Read the model definition and answer for the solid it produces. Units are mm, in the model's axes. Round coordinates to 2 decimals unless told otherwise and drop trailing zeros. Write each loop counter-clockwise with the first axis right and the second up, starting at its lowest first coordinate (ties: lowest second). Pieces come first, ordered by that corner, then holes. Notation, with made-up numbers: (45, 10) - (86, 10) arc R29 ccw to (86, 31) - close; hole circle Ø2 at (2, 50). An arc over 180 degrees is marked (long way). Answer as CSV lines item,"result". Start each with the question number.
1) Each of these flat-tipped pins is pushed along its axis until it touches: pin 1 (1 mm diameter, centred on x = 14.5, y = -9.5, fed in from -Z); pin 2 (5 mm diameter, centred on x = 5, y = -6, fed in from -Z); pin 3 (12 mm diameter, centred on x = 13.5, z = 14.5, fed in from +Y). Where does it stop, or does it pass through?
2) Find section B-B on y = -12. Determine the outline of the cut face in (x, z).
3) For a pull along Y with two mould halves and no side action, classify faces 1 (the cylindrical face through (-2.2, -30.16, 25.2)), 2 (the flat face through (0.267, -12.833, 23.55)), 3 (the flat face through (0, -36, 0)) as +Y half, -Y half, draft (parallel to the pull), parting line (faces both ways), or undercut.
4) Consider line 1 along X through (y, z) = (-18, 20); line 2 along Y through (x, z) = (3.5, 27); line 3 along X through (y, z) = (-18.5, 22.5). Determine where each line is inside the solid, lowest interval first.
5) Find section A-A on x = 13.5. Determine the outline of the cut face in (y, z), then the cut area to 3 significant figures.
from build123d import *

# Parameters (mm, degrees)
F1_DEPTH      = 38.1
F3_DEPTH      = 19.051
F3_DEPTH_BACK = 19.051
F4_R          = 4.7625
F5_DEPTH      = 28.5749043881


with BuildPart() as f1:
    # F0 (on Front) → F1 (new body)
    with BuildSketch(Plane.XZ):
        Polygon((-19.05, 38.1), (-19.05, 0), (0, 0), (19.05, 0), (19.05, 38.1), align=None)
    extrude(amount=F1_DEPTH)

    # F2 (on Right) → F3 (cut, two sides)
    with BuildSketch(Plane.YZ) as f3_sk:
        Polygon((-33.6039864189, 0), (0, 0), (0, 38.1), align=None)
    extrude(amount=-F3_DEPTH, mode=Mode.SUBTRACT)
    extrude(f3_sk.sketch, amount=F3_DEPTH_BACK, mode=Mode.SUBTRACT)

    # F4 (on face) → F5 (cut, through all)
    with BuildSketch(Plane(origin=(0, -18.9007929031, 16.6703933864), x_dir=(-1, 0, 0), z_dir=(0, 0.7499712438, -0.6614704328))):
        with Locations((0, 3.1729304735)):
            Circle(F4_R)
    extrude(amount=-F5_DEPTH, mode=Mode.SUBTRACT)


solid = f1.part
Check values:
1,pin 1,"stops at z = 26.76"
1,pin 2,"stops at z = 28.46"
1,pin 3,"stops at y = -15.52"
2,outline,"(-19.05, 24.49) - (19.05, 24.49) - (19.05, 38.1) - (-19.05, 38.1) - close"
3,face 1,"undercut"
3,face 2,"+Y half"
3,face 3,"draft"
4,line 1,"x = -19.05 to -4.76, 4.76 to 19.05"
4,line 2,"y = -38.1 to -30.7, -20.93 to -9.79"
4,line 3,"x = -19.05 to -4.53, 4.53 to 19.05"
5,outline,"(-38.1, 0) - (-33.6, 0) - (0, 38.1) - (-38.1, 38.1) - close"
5,area,"811 mm^2"
